```python
from build123d import *

# Parameters (mm, degrees)
ESQUISSE2_W               = 198
ESQUISSE2_H               = 1
T_LE_DE_BASE_PLI_E1_DEPTH = 203.5
ESQUISSE7_R               = 2
ENL_V_MAT_EXTRU_1_DEPTH   = 227.305656138
ENL_V_MAT_EXTRU_2_DEPTH   = 227.305656138


# Sheet-metal steps are written as plain solids
with BuildPart() as part:
    # Esquisse2 → Tôle de base pliée1 (new body)
    with BuildSketch(Plane(origin=(0, 0, 0), x_dir=(1, 0, 0), z_dir=(0, 1, 0))):
        with Locations((0, -0.5)):
            Rectangle(ESQUISSE2_W, ESQUISSE2_H)
    extrude(amount=T_LE_DE_BASE_PLI_E1_DEPTH)

    # Esquisse7 → Enlèv. mat.-Extru.1 (cut, through all)
    with BuildSketch(Plane.XY.offset(1)):
        with Locations((-90, 194.5)):
            Circle(ESQUISSE7_R)
        with Locations((90, 194.5)):
            Circle(ESQUISSE7_R)
        with Locations((-90, 8.82)):
            Circle(ESQUISSE7_R)
        with Locations((90, 8.82)):
            Circle(ESQUISSE7_R)
        with Locations((-45.7, 34.51)):
            Circle(ESQUISSE7_R)
        with Locations((45.7, 34.51)):
            Circle(ESQUISSE7_R)
        with Locations((-30, 68.5)):
            Circle(ESQUISSE7_R)
        with Locations(Location((30, 68.5, 0), (0, 0, 180))):
            Circle(ESQUISSE7_R)
    extrude(amount=-ENL_V_MAT_EXTRU_1_DEPTH, mode=Mode.SUBTRACT)

    # Esquisse10 → Enlèv. mat.-Extru.2 (cut, through all)
    with BuildSketch(Plane.XY.offset(1)):
        Polygon((-74, 0), (-20.7, 24.51), (20.7, 24.51), (74, 0), align=None)
    extrude(amount=-ENL_V_MAT_EXTRU_2_DEPTH, mode=Mode.SUBTRACT)


solid = part.part
```
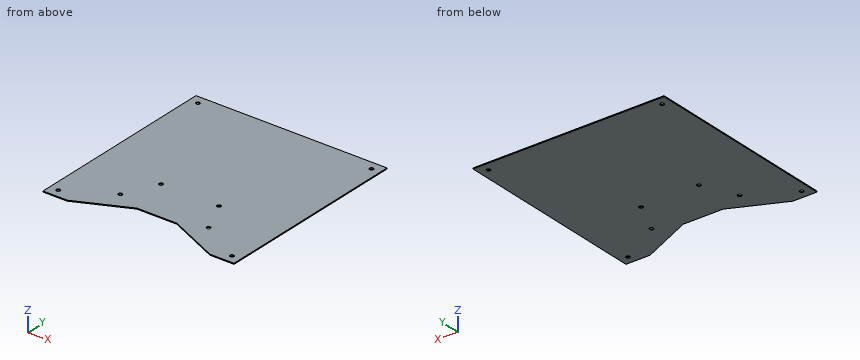
Can you work these out from the model? Positions are in its coordinate system, mm. Coordinates: 2 decimals unless noted, no trailing zeros. Order: outer loops, then holes, each group sorted by start corner. A loop starts at its lowest first (then second) coordinate and runs counter-clockwise, first axis right, second up.
1. I'm going to push a flat-ended pin straight in: pin 1 (2.5 mm diameter, centred on x = -90, y = 194.5, fed in from -Z). Where does the tip first touch, or does it pass through?
2. If we section it at C-C (x = -54): Please give me the cut outline in (y, z), then the cut area to 3 significant figures.
3. If we section it at B-B (x = -14.5): Please give me the cut outline in (y, z).
4. If we section it at A-A (z = 0.4): Give the number of separate pieces and of enclosed holes in the cut face, then the cut area to 3 significant figures.
5. I need wall thicknesses on line 1 (Y direction, x = 90, z = 0.75); line 2 (Y direction, x = -91, z = 0.25); line 3 (Y direction, x = -30, z = 0.4). Which ranges of each line are inside material? Lowest first, please.
Entries:
1. pin 1: passes through
2. outline: (9.2, 0) - (203.5, 0) - (203.5, 1) - (9.2, 1) - close
2. area: 194 mm2
3. outline: (24.51, 0) - (203.5, 0) - (203.5, 1) - (24.51, 1) - close
4. separate pieces: 1
4. enclosed holes: 8
4. area: 37,900 mm2
5. line 1: y = 0 to 6.82, 10.82 to 192.5, 196.5 to 203.5
5. line 2: y = 0 to 7.09, 10.55 to 192.77, 196.23 to 203.5
5. line 3: y = 20.23 to 66.5, 70.5 to 203.5
